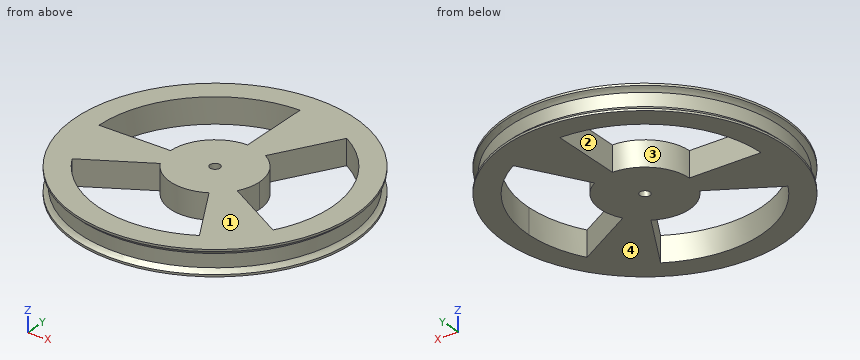
```python
from build123d import *

# Parameters (mm, degrees)
ESBO_O1_R                = 27.5
RESSALTO_EXTRUS_O1_DEPTH = 5
ESBO_O9_R                = 1
CORTE_EXTRUS_O1_DEPTH    = 5
CORTE_EXTRUS_O2_DEPTH    = 5


# Read off the part's stored shape, not the designer's step: Corte-Revolu__o4
with BuildPart() as part:
    # Esbo_o1 → Ressalto-extrus_o1 (new body)
    with BuildSketch(Plane.XY):
        Circle(ESBO_O1_R)
    extrude(amount=RESSALTO_EXTRUS_O1_DEPTH)

    # Corte-Revolu_o4 outline → Corte-Revolu_o4 (revolve, cut)
    with BuildSketch(Plane.XZ):
        with BuildLine():
            Line((27.5, 0.405836604), (27.5, 4.594163396))
            ThreePointArc((27.5, 4.594163396), (27.026509852, 4.253637489), (26.649701973, 3.808478377))
            Line((26.649701973, 3.808478377), (26.649701973, 1.191521623))
            ThreePointArc((26.649701973, 1.191521623), (27.026509852, 0.746362511), (27.5, 0.405836604))
        make_face()
    revolve(axis=Axis((0, 0, 0), (0, 0, 1)), mode=Mode.SUBTRACT)

    # Esbo_o9 → Corte-extrus_o1 (cut)
    with BuildSketch(Plane.XY.offset(5)):
        Circle(ESBO_O9_R)
    extrude(amount=-CORTE_EXTRUS_O1_DEPTH, mode=Mode.SUBTRACT)

    # Esbo_o10 → Corte-extrus_o2 (cut)
    with BuildSketch(Plane.XY.offset(5)):
        with BuildLine():
            ThreePointArc((-8.8, 0), (-6.222539674, 6.222539674), (0, 8.8))
            Line((0, 8.8), (0, 23))
            ThreePointArc((0, 23), (-16.263455967, 16.263455967), (-23, 0))
            Line((-23, 0), (-8.8, 0))
        make_face()
        with BuildLine():
            Line((11.5, 19.918584287), (4.4, 7.621023553))
            ThreePointArc((4.4, 7.621023553), (7.621023553, 4.4), (8.8, 0))
            ThreePointArc((8.8, 0), (8.500147271, -2.277607597), (7.621023553, -4.4))
            Line((7.621023553, -4.4), (19.918584287, -11.5))
            ThreePointArc((19.918584287, -11.5), (22.216294005, -5.952838037), (23, 0))
            ThreePointArc((23, 0), (19.918584287, 11.5), (11.5, 19.918584287))
        make_face()
        with BuildLine():
            ThreePointArc((4.4, -7.621023553), (-2.277607597, -8.500147271), (-7.621023553, -4.4))
            Line((-7.621023553, -4.4), (-19.918584287, -11.5))
            ThreePointArc((-19.918584287, -11.5), (-5.952838037, -22.216294005), (11.5, -19.918584287))
            Line((11.5, -19.918584287), (4.4, -7.621023553))
        make_face()
    extrude(amount=-CORTE_EXTRUS_O2_DEPTH, mode=Mode.SUBTRACT)


solid = part.part
```
Design review of the part built by this model. Coordinates are the model's own, in mm. Face numbers are marked on the shaded views. A direction names the side the tool comes from. Give positions to 0.01 mm unless a question says otherwise; leave off trailing zeros. Write each loop counter-clockwise with the first axis right and the second up, starting at its lowest first coordinate (ties: lowest second). Pieces come first, ordered by that corner, then holes. Notation, with made-up numbers: (-31, 60.5) - (-23, 60.5) arc R22 ccw to (-23, 89.5) - close; hole circle Ø3 at (60, -13). An arc over 180 degrees is marked (long way). Return JSON: item names as keys, results as strings. Group by question number.
(1) Machinability: for the marked faces 1 and 2, which of the approach directions +Z, -Z, +X, -X, +Y, -Y give a long, thin tool a straight path to every point of the face, cutting with its end or side? Answer none if there is none.
(2) To check wall thickness, follow probe 1 along Y at (x, z) = (-8, 3.8); probe 2 along X at (y, z) = (11, 2.2); probe 3 along Y at (x, z) = (6.5, 4). State the ranges of each line that lie inside material, in increasing order.
(3) Insertion check: pin 1 (1.5 mm diameter, centred on x = -21.5, y = 4.5, fed in from +Z); pin 2 (1.5 mm diameter, centred on x = -17, z = 3.5, fed in from +Y); pin 3 (1 mm diameter, centred on y = 18, z = 1.5, fed in from -X); pin 4 (3 mm diameter, centred on y = 7, z = 2.5, fed in from +X). Each pin has a flat end and moves straight along its axis. Give the tip position at first contact, or say it passes through.
(4) We need section A-A, the plane z = 2.7. Give the boundary of the cut face in (x, y).
(5) Mouldability with a two-part tool opening along Y and no side actions: class the marked faces 3 and 4 as +Y half, -Y half, draft (parallel to the pull), parting line (faces both ways), or undercut.
(6) We need section B-B, the plane y = 5. Give the number of separate pieces and of enclosed holes in the cut face, then the cut area to 3 significant figures.
Reported:
{
 "1": {"face 1": "+Z, +X, -X, +Y, -Y", "face 2": "+Z, -Z"},
 "2": {"probe 1": "y = -25.42 to -21.56, -4.62 to 3.67, 21.56 to 25.42", "probe 2": "x = -24.27 to -20.2, 0 to 6.35, 20.2 to 24.27", "probe 3": "y = -25.99 to -22.06, -11.26 to 5.93, 11.26 to 25.99"},
 "3": {"pin 1": "passes through", "pin 2": "stops at y = 21.18", "pin 3": "stops at x = -20.1", "pin 4": "stops at x = 26.08"},
 "4": {"outline": "circle Ø53.3 at (0, 0); hole (-23, 0) - (-8.8, 0) arc R8.8 cw to (0, 8.8) - (0, 23) arc R23 ccw to start; hole (-19.92, -11.5) arc R23 ccw to (11.5, -19.92) - (4.4, -7.62) arc R8.8 cw to (-7.62, -4.4) - close; hole circle Ø2 at (0, 0); hole (4.4, 7.62) arc R8.8 cw to (7.62, -4.4) - (19.92, -11.5) arc R23 ccw to (11.5, 19.92) - close"},
 "5": {"face 3": "undercut", "face 4": "draft"},
 "6": {"separate pieces": "3", "enclosed holes": "0", "area": "112 mm2"}
}
